from build123d import *

# Parameters (mm, degrees)
CROQUIS1_W              = 60
CROQUIS1_H              = 40
SALIENTE_EXTRUIR1_DEPTH = 80
REDONDEO1_R             = 10
CROQUIS2_R              = 12.5
SALIENTE_EXTRUIR2_DEPTH = 40


with BuildPart() as part:
    # Croquis1 → Saliente-Extruir1 (new body)
    with BuildSketch(Plane.XY):
        Rectangle(CROQUIS1_W, CROQUIS1_H)
    extrude(amount=SALIENTE_EXTRUIR1_DEPTH)

    # Redondeo1
    redondeo1_edges = [part.edges().sort_by_distance(p)[0] for p in [
        (-30, 0, 80),
        (30, 0, 80),
    ]]
    fillet(redondeo1_edges, radius=REDONDEO1_R)

    # Croquis2 → Saliente-Extruir2 (add)
    with BuildSketch(Plane.XZ.offset(20)):
        with Locations(Location((0, 55, 0), (0, 0, 90))):
            Circle(CROQUIS2_R)
    extrude(amount=SALIENTE_EXTRUIR2_DEPTH)


solid = part.part
Check sheet for the modelled part. Datum: model origin and axes. Units: mm. A direction names the side the tool comes from. Round coordinates to 2 decimals unless told otherwise and drop trailing zeros. Loops run counter-clockwise (first coordinate to the right, second up) from the corner with the lowest first, then second, coordinate; pieces in that order, holes last. Notation, with made-up numbers: M -5.75,-11.5 L 3.25,-11.5 A26 ccw 3.25,14.5 Z; hole C 89.25,5.25 d11. An arc over 180 degrees is marked long. One line per question, with ' | ' between items. Start each with the question number.
Item 1: Gauge pin test, flat ends, axial feed: pin 1 Ø10 at (x, z) = (-5, 26) entering from -Y; pin 2 Ø4 at (x, y) = (-12.5, -39) entering from -Z. Record the tip position at first contact, or that the pin passes through.
Item 2: Set-up check for faces 1 (the face through (0, -60, 55)), 2 (the face through (-8.45, -39.72, 45.79)): record each of +Z, -Z, +X, -X, +Y, -Y from which the full face is reachable in a straight line by a thin tool's end or side.
Item 3: Release check for a two-part mould opening along Y. For faces 3 (the face through (-27.15, 0.28, 76.99)), 4 (the face through (0, -20, 39)), 5 (the face through (0, 20, 39)) record: released by +Y, released by -Y, zero draft, split by the parting line, or undercut.
Item 4: Section check A-A (z = 55). Record the boundary of the cut face in (x, y), and give its area (3 significant figures).
Item 5: Section check B-B (x = 0). Record the boundary of the cut face in (y, z), and give its area (3 significant figures).
Item 6: Section check D-D (z = 35.5). Record the boundary of the cut face in (x, y).
Item 7: Scan lines: probe 1 along Y at (x, z) = (21.5, 31.5); probe 2 along X at (y, z) = (-30, 44.5); probe 3 along Z at (x, y) = (-8, -21). Record each from-to range of solid material in increasing order.
Item 8: Section check C-C (y = -26.5). Record the boundary of the cut face in (x, z), and give its area (3 significant figures).
Worked out:
1) pin 1: y = -20 | pin 2: z = 48.22
2) face 1: +Z, -Z, +X, -X, -Y | face 2: -Y
3) face 3: zero draft | face 4: released by -Y | face 5: released by +Y
4) outline: M -30,-20 L -12.5,-20 L -12.5,-60 L 12.5,-60 L 12.5,-20 L 30,-20 L 30,20 L -30,20 Z | area: 3,400 mm^2
5) outline: M -60,42.5 L -20,42.5 L -20,0 L 20,0 L 20,80 L -20,80 L -20,67.5 L -60,67.5 Z | area: 4,200 mm^2
6) outline: M -30,-20 L 30,-20 L 30,20 L -30,20 Z
7) probe 1: -20 to 20 | probe 2: -6.78 to 6.78 | probe 3: 45.4 to 64.6
8) outline: C 0,55 d25 | area: 491 mm^2
